Autodesk Inventor part; units mm, degrees
ref_plane "IDS_WORKPLANE{1}" through (-13.2334, 0, 0) normal (1, 0, 0) x (0, 0, -1)
ref_plane "Work Plane2" through (41.275, 0, 0) normal (0, 0, -1) x (1, 0, 0)
ref_plane "YZ Plane" through (0, 0, 0) normal (1, 0, 0) x (0, 1, 0)
sketch "Sketch1" plane through (0, 0, 0) normal (0, 0, 1) x (1, 0, 0)
  line L0 (-13.2334, 0) -> (57.15, 0)
  line L1 (57.15, 0) -> (57.15, 7.9375)
  line L2 (57.15, 7.9375) -> (19.05, 7.9375)
  line L3 (19.05, 7.9375) -> (17.6644, 7.9375)
  line L4 (17.6644, 7.9375) -> (0, 7.9375)
  line L5 (0, 7.9375) -> (0, 11.1125)
  line L6 (-28.1879, 0) -> (71.373, 0)
  line L7 (0, -2.2617) -> (0, 13.5702)
  line L8 (0, 11.1125) -> (-10.2558, 11.1125)
  arc A0 (-10.2558, 11.1125) -> (-13.2334, 0) centre (8.9916, 0) ccw
  line L9 (19.05, 7.9375) -> (0, 7.9375) construction
  dimension "d0" = 57.15
  dimension "d1" = 38.1
  dimension "d2" = 1.3856
  dimension "d3" = 13.2334
  dimension "d4" = 15.875
  dimension "d5" = 15.875
  dimension "d9" = 22.225
  dimension "d10" = 0
  dimension "d13" = 22.225
revolve "Body" add sketch "Sketch1" angle 360 about axis through (-13.2334, 0, 0) along (1, 0, 0)
ref_plane "IDS_WORKPLANE{1}" through (-13.2334, 0, 0) normal (1, 0, 0) x (0, 0, -1)
sketch "Sketch2" plane through (-13.2334, 0, 0) normal (1, 0, 0) x (0, 0, -1)
  circle A0 centre (0, 0) radius 11.1125
  line L0 (0, -15.5575) -> (0, 15.5575)
  line L1 (15.5575, 0) -> (-15.5575, 0)
  line L2 (-11.1125, 1.6891) -> (11.1125, 1.6891)
  line L3 (11.1125, 1.6891) -> (11.1125, -1.6891)
  line L4 (11.1125, -1.6891) -> (-11.1125, -1.6891)
  line L5 (-11.1125, -1.6891) -> (-11.1125, 1.6891)
  line L6 (-11.1125, 0) -> (11.1125, 0) construction
  line L7 (0, 1.6891) -> (0, -1.6891) construction
  dimension "d15" = 3.3782
extrude "Slot" cut sketch "Sketch2" along normal blind 6.0706 contours L1 L0 L2 A0 | L3 L4 A0 | A0 L4 L0 L1 | A0 L2 L3 | L1 A0 L2 L0 | L0 L4 A0 L1 | L5 L2 A0 | A0 L4 L5
thread "Thread"
sketch "Sketch3" plane through (0, 0, 0) normal (0, 0, 1) x (1, 0, 0)
  line L0 (57.15, 0) -> (57.15, 7.9375)
  line L1 (57.15, 7.9375) -> (19.05, 7.9375)
  line L2 (-13.2334, 0) -> (57.15, 0)
  arc A0 (57.15, 0) -> (55.0232, 7.9375) centre (41.275, 0) ccw
  line L3 (57.15, -7.9375) -> (57.15, 7.9375)
  line L4 (55.0232, 7.9375) -> (55.0232, 0)
  line L5 (55.0232, 0) -> (57.15, 0)
  dimension "d40" = 15.875
revolve "Fillet1" cut sketch "Sketch3" angle 360 about axis through (-13.2334, 0, 0) along (1, 0, 0) contours A0 L1 L0
chamfer "Chamfer" distance 1.1545 angle 45 1 edges at (55.0232, -7.9375, 0)
ref_plane "Work Plane2" through (41.275, 0, 0) normal (0, 0, -1) x (1, 0, 0)
fillet "Fillet4" radius 1.5748 1 edges at (0, -7.9375, 0)
equation "\"d0\" = NLG"
equation "\"d1\" = GEL"
equation "\"d2\" = GAL"
equation "\"d3\" = KOH"
equation "\"d4\" = GD"
equation "\"d5\" = BDM"
equation "\"d9\" = KOD"
equation "\"d13\" = KR"
equation "\"d15\" = SBR"
equation "\"d16\" = STI"
equation "\"d40\" = GD"
equation "\"d46\" = R"
equation "\"d11\" = GEL"
equation "\"d43\" = 0.5 * RR"
equation "\"GD\" = NND"
equation "\"NLG\" = 57.15"
equation "\"GEL\" = 38.1"
equation "\"KOD\" = 22.225"
equation "\"KOH\" = 13.2334"
equation "\"GAL\" = 1.38557"
equation "\"BDM\" = NND"
equation "\"SBR\" = 3.3782"
equation "\"STI\" = 6.0706"
equation "\"KEWI\" = 0"
equation "\"KR\" = KOD"
equation "\"d14\" = -KOH"
equation "\"R\" = 1.5748"
equation "\"THREADDIA\" = 15.875"
equation "\"TOA\" = 30deg"
equation "\"KOH1\" = 10.7188"
equation "\"NND\" = 15.875"
equation "\"GD1\" = 13.12672"
equation "\"THREADDESC\" = 1.2345"
properties part number "ANSI B18.6.2 - 5/8-11 UNC - 2.25, SFHCSI" material "Steel, Mild"
The model under review builds one solid part; all positions refer to its coordinate system, in mm. A direction names the side the tool comes from. Round coordinates to 2 decimals unless told otherwise and drop trailing zeros. Loops run counter-clockwise (first coordinate to the right, second up) from the corner with the lowest first, then second, coordinate; pieces in that order, holes last. Notation, with made-up numbers: M -1.5,10 L 15.5,10 A25 ccw 15.5,43 Z; hole C 32.25,53 d7. An arc over 180 degrees is marked long. Answer as CSV lines item,"result". Start each with the question number.
Item 1: For faces 4 (the face through (-5.2, -2.41, 10.85)), 5 (the face through (-10, 1.689, 0)), list the 3-axis set-ups (+Z, -Z, +X, -X, +Y, -Y) from which the entire face can be reached by the end or side of a thin tool; tool diameter is ignored.
Item 2: Mouldability with a two-part tool opening along Y and no side actions: class faces 1 (the face through (27.36, -1.72, 7.75)), 2 (the face through (0, -5, 8.3)), 3 (the face through (-7.163, 0, 0)) as released by +Y, released by -Y, zero draft, split by the parting line, or undercut.
Item 3: Consider section A-A (x = 26). Write out the cut boundary in (y, z) (1 decimal), then the cut area to 3 significant figures.
Item 4: Insertion check: P1, Ø6.5, axis at x = -10, z = -5, coming from the +Y side; P2, Ø1.7, axis at y = 0, z = 0, coming from the -X side; P3, Ø1.5, axis at y = -0.5, z = 2.5, coming from the +X side. Each pin has a flat end and moves straight along its axis. Give the tip position at first contact, or say it passes through.
Item 5: Wall thickness on line 1 (Y direction, x = 22, z = -0.5); line 2 (Y direction, x = -6, z = -1.75): over which ranges is each line inside the solid? List them lowest first. Write a range as [from, to].
Answer:
1,face 4,"+X, -X"
1,face 5,"+Z, -Z, -X"
2,face 1,"split by the parting line"
2,face 2,"zero draft"
2,face 3,"undercut"
3,outline,"C 0,0 d15.9"
3,area,"198 mm^2"
4,P1,"stops at y = 10.97"
4,P2,"stops at x = -7.16"
4,P3,"stops at x = 57.05"
5,line 1,"y = [-7.92, 7.92]"
5,line 2,"y = [-10.97, 10.97]"
